For this review, use the dimensioned drawing (mm, ordinates from the lowest corner) and the shaded views. A direction names the side the tool comes from. Coordinates: 2 decimals unless noted, no trailing zeros. Loops run counter-clockwise (first coordinate to the right, second up) from the corner with the lowest first, then second, coordinate; pieces in that order, holes last. Notation, with made-up numbers: (88.5, 69.25) - (101.5, 69.25) arc R19 cw to (101.5, 80.25) - close; hole circle Ø6 at (14.5, 5.25). An arc over 180 degrees is marked (long way). Return JSON: item names as keys, results as strings. Group by question number.
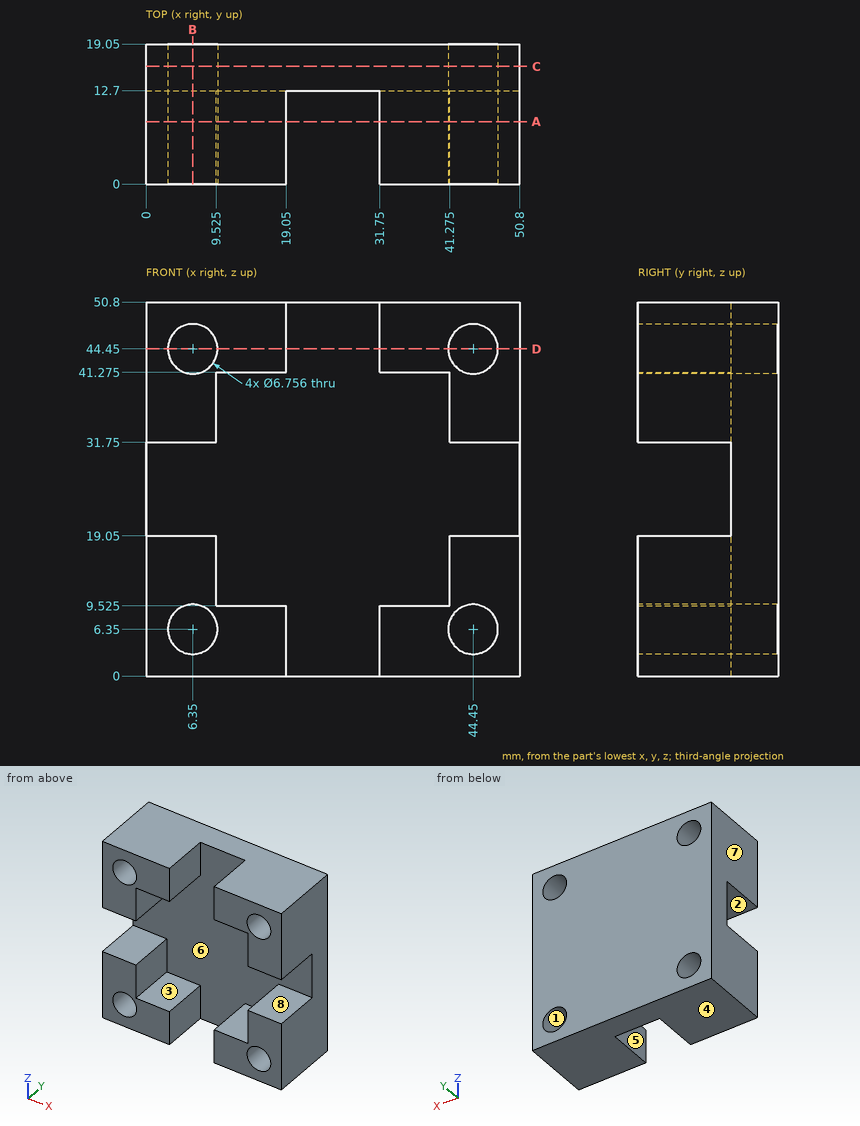
Item 1: Add section C-C (y = 16). State the section outline as (x, z) points, then the cut area to 3 significant figures.
Item 2: Add section B-B (x = 6.35). State the section outline as (y, z) points, then the cut area to 3 significant figures.
Item 3: To check wall thickness, follow line 1 (X direction, y = 5, z = 44.45); line 2 (Z direction, x = 34, y = 11) (1 decimal). State the ranges of each line that lie inside material, in increasing order. Write a range as from..to.
Item 4: For P1, Ø6, axis at x = 41.5, y = 14, coming from the -Z side; P2, Ø1.5, axis at x = 29.5, z = 6, coming from the -Y side, all flat-tipped, find the tip position at first contact; note any pin that passes through.
Item 5: Draft analysis for pull direction X (two halves, no side actions). For the marked faces 6, 7 and 8, state which applies: pulls with the +X half, pulls with the -X half, needs draft (parallel to the pull), parting line crosses it, or undercut.
Item 6: Add section D-D (z = 44.45). State the section outline as (x, y) points, then the cut area to 3 significant figures.
Item 7: Add section A-A (y = 8.5). Give the number of separate pieces and of enclosed holes in the cut face.
Item 8: For the marked faces 1, 2, 3, 4 and 5, list the 3-axis set-ups (+Z, -Z, +X, -X, +Y, -Y) from which the entire face can be reached by the end or side of a thin tool; tool diameter is ignored.
Answers below:
{
 "1": {"outline": "(0, 0) - (50.8, 0) - (50.8, 50.8) - (0, 50.8) - close; hole circle Ø6.76 at (6.35, 6.35); hole circle Ø6.76 at (6.35, 44.45); hole circle Ø6.76 at (44.45, 6.35); hole circle Ø6.76 at (44.45, 44.45)", "area": "2,440 mm^2"},
 "2": {"outline": "(0, 0) - (19.05, 0) - (19.05, 2.97) - (0, 2.97) - close; (0, 9.73) - (19.05, 9.73) - (19.05, 41.07) - (0, 41.07) - (0, 31.75) - (12.7, 31.75) - (12.7, 19.05) - (0, 19.05) - close; (0, 47.83) - (19.05, 47.83) - (19.05, 50.8) - (0, 50.8) - close", "area": "549 mm^2"},
 "3": {"line 1": "x = 0..2.97, 9.73..19.05, 31.75..41.07, 47.83..50.8", "line 2": "z = 0..9.5, 41.3..50.8"},
 "4": {"P1": "stops at z = 0", "P2": "stops at y = 12.7"},
 "5": {"face 6": "undercut", "face 7": "pulls with the -X half", "face 8": "needs draft"},
 "6": {"outline": "(0, 0) - (2.97, 0) - (2.97, 19.05) - (0, 19.05) - close; (9.73, 0) - (19.05, 0) - (19.05, 12.7) - (31.75, 12.7) - (31.75, 0) - (41.07, 0) - (41.07, 19.05) - (9.73, 19.05) - close; (47.83, 0) - (50.8, 0) - (50.8, 19.05) - (47.83, 19.05) - close", "area": "549 mm^2"},
 "7": {"separate pieces": "4", "enclosed holes": "4"},
 "8": {"face 1": "+Y, -Y", "face 2": "+X, -X, -Y", "face 3": "-Y", "face 4": "-Z, +X, -X, +Y, -Y", "face 5": "+Z, -Z, -Y"}
}
